```python
from build123d import *

# Parameters (mm, degrees)
SKETCH1_R               = 2
SKETCH1_R_2             = 13
BOSS_EXTRUDE1_DEPTH     = 80
CUT_EXTRUDE1_DEPTH      = 75
CUT_EXTRUDE2_DEPTH      = 99.05738116
CUT_EXTRUDE2_DEPTH_BACK = 99.05738116
SKETCH3_R               = 1.5
FILLET3_R               = 2
FILLET2_R               = 3


with BuildPart() as part:
    # Sketch1 → Boss-Extrude1 (new body)
    with BuildSketch(Plane.XY):
        with BuildLine():
            Line((-25, 0), (-25, -20))
            Line((-25, -20), (-34.5, -20))
            Line((-34.5, -20), (-34.5, -25))
            Line((-34.5, -25), (34.5, -25))
            Line((34.5, -25), (34.5, -20))
            Line((34.5, -20), (25, -20))
            Line((25, -20), (25, 0))
            ThreePointArc((25, 0), (0, 25), (-25, 0))
        make_face()
        with Locations((-12.40972401, 12.40972401)):
            Circle(SKETCH1_R, mode=Mode.SUBTRACT)
        with Locations((12.40972401, 12.40972401)):
            Circle(SKETCH1_R, mode=Mode.SUBTRACT)
        with Locations((12.40972401, -12.40972401)):
            Circle(SKETCH1_R, mode=Mode.SUBTRACT)
        with Locations((-12.40972401, -12.40972401)):
            Circle(SKETCH1_R, mode=Mode.SUBTRACT)
        Circle(SKETCH1_R_2, mode=Mode.SUBTRACT)
    extrude(amount=BOSS_EXTRUDE1_DEPTH)

    # Sketch2 → Cut-Extrude1 (cut)
    with BuildSketch(Plane.XY.offset(80)):
        with BuildLine():
            Line((-23, 0), (-23, -25))
            Line((-23, -25), (23, -25))
            Line((23, -25), (23, 0))
            ThreePointArc((23, 0), (0, 23), (-23, 0))
        make_face()
    extrude(amount=-CUT_EXTRUDE1_DEPTH, mode=Mode.SUBTRACT)

    # Sketch3 → Cut-Extrude2 (cut, two sides: drawn at the far end of the back side and taken through both)
    with BuildSketch(Plane(origin=(0, -20, 0), x_dir=(1, 0, 0), z_dir=(0, 1, 0)).offset(-CUT_EXTRUDE2_DEPTH_BACK)):
        with Locations(Location((29.5, -40, 0), (0, 0, 270))):
            Circle(SKETCH3_R)
        with Locations(Location((29.5, -60, 0), (0, 0, 270))):
            Circle(SKETCH3_R)
        with Locations(Location((29.5, -20, 0), (0, 0, 270))):
            Circle(SKETCH3_R)
        with Locations(Location((-29.5, -60, 0), (0, 0, 90))):
            Circle(SKETCH3_R)
        with Locations(Location((-29.5, -40, 0), (0, 0, 90))):
            Circle(SKETCH3_R)
        with Locations(Location((-29.5, -20, 0), (0, 0, 90))):
            Circle(SKETCH3_R)
    extrude(amount=CUT_EXTRUDE2_DEPTH + CUT_EXTRUDE2_DEPTH_BACK, mode=Mode.SUBTRACT)

    # Fillet3
    fillet3_edges = [part.edges().sort_by_distance(p)[0] for p in [
        (25, -20, 40),
        (-25, -20, 40),
    ]]
    fillet(fillet3_edges, radius=FILLET3_R)

    # Fillet2
    fillet2_edges = [part.edges().sort_by_distance(p)[0] for p in [
        (-34.5, -22.5, 0),
        (-34.5, -22.5, 80),
        (34.5, -22.5, 80),
        (34.5, -22.5, 0),
    ]]
    fillet(fillet2_edges, radius=FILLET2_R)


solid = part.part
```
Input: part model. Units: mm. Frame: model coordinates. A direction names the side the tool comes from. Give positions to 0.01 mm unless a question says otherwise; leave off trailing zeros. Order: outer loops, then holes, each group sorted by start corner. A loop starts at its lowest first (then second) coordinate and runs counter-clockwise, first axis right, second up.
1. Cut plane A-A (x = 0). Return loops of the section in (y, z).
Computed:
outline: (-25, 0) - (-13, 0) - (-13, 5) - (-25, 5) - close; (13, 0) - (25, 0) - (25, 80) - (23, 80) - (23, 5) - (13, 5) - close
2. Cut plane D-D (x = 29.5). Return loops of the section in (y, z), and give its area (3 significant figures).
Computed:
outline: (-25, 0) - (-20, 0) - (-20, 18.5) - (-25, 18.5) - close; (-25, 21.5) - (-20, 21.5) - (-20, 38.5) - (-25, 38.5) - close; (-25, 41.5) - (-20, 41.5) - (-20, 58.5) - (-25, 58.5) - close; (-25, 61.5) - (-20, 61.5) - (-20, 80) - (-25, 80) - close
area: 355 mm2
3. Set-up query: faces 1 (the face through (-10.316, -7.91, 2.465)), 2 (the face through (23, -13, 43)), 3 (the face through (-32, -20, 39)). Return all of +Z, -Z, +X, -X, +Y, -Y with unobstructed straight access to the full face (end or side cutting, diameter ignored); none if empty.
Computed:
face 1: +Z, -Z
face 2: +Z, -Y
face 3: +Z, -Z, -X, +Y
4. Line query: probe 1 along Y at (x, z) = (0, 1.8); probe 2 along X at (y, z) = (-23, 15.5); probe 3 along Z at (x, y) = (-29, -22). Output: solid intervals per line, ascending.
Computed:
probe 1: y = -25 to -13, 13 to 25
probe 2: x = -34.5 to -23, 23 to 34.5
probe 3: z = 0 to 18.59, 21.41 to 38.59, 41.41 to 58.59, 61.41 to 80
5. Pin query (flat end, axial travel): pin 1 Ø20 at (y, z) = (-6.5, 34.5) entering from +X; pin 2 Ø4 at (x, z) = (31, 52.5) entering from +Y; pin 3 Ø14.5 at (y, z) = (-9.5, 36.5) entering from -X. Return the tip coordinate at first contact, or that it passes through.
Computed:
pin 1: stops at x = 25
pin 2: stops at y = -20
pin 3: stops at x = -25
6. Cut plane B-B (y = -21). Return loops of the section in (x, z).
Computed:
outline: (-34.5, 3) arc R3 ccw to (-31.5, 0) - (31.5, 0) arc R3 ccw to (34.5, 3) - (34.5, 77) arc R3 ccw to (31.5, 80) - (23, 80) - (23, 5) - (-23, 5) - (-23, 80) - (-31.5, 80) arc R3 ccw to (-34.5, 77) - close; hole circle Ø3 at (-29.5, 20); hole circle Ø3 at (-29.5, 40); hole circle Ø3 at (-29.5, 60); hole circle Ø3 at (29.5, 20); hole circle Ø3 at (29.5, 40); hole circle Ø3 at (29.5, 60)
7. Cut plane C-C (z = 20). Return loops of the section in (x, y), and give its area (3 significant figures).
Computed:
outline: (-34.5, -25) - (-31, -25) - (-31, -20) - (-34.5, -20) - close; (-28, -25) - (-23, -25) - (-23, 0) arc R23 cw to (23, 0) - (23, -25) - (28, -25) - (28, -20) - (27, -20) arc R2 cw to (25, -18) - (25, 0) arc R25 ccw to (-25, 0) - (-25, -18) arc R2 cw to (-27, -20) - (-28, -20) - close; (31, -25) - (34.5, -25) - (34.5, -20) - (31, -20) - close
area: 318 mm2
8. Draft query along Y for faces 4 (the face through (-14.408, -12.322, 2.465)), 5 (the face through (32, -20, 39)), 6 (the face through (-23, -12, 43)), 7 (the face through (14.257, -13.176, 2.465)). Return one class per face: released by +Y, released by -Y, zero draft, split by the parting line, or undercut.
Computed:
face 4: undercut
face 5: released by +Y
face 6: zero draft
face 7: undercut
